Input: dimensioned drawing with shaded views. Units: mm. Origin: part minimum x, y, z. A direction names the side the tool comes from. Round coordinates to 2 decimals unless told otherwise and drop trailing zeros. Loops run counter-clockwise (first coordinate to the right, second up) from the corner with the lowest first, then second, coordinate; pieces in that order, holes last. Notation, with made-up numbers: M 51,-4.5 L 67,-4.5 A15 ccw 67,19.5 Z; hole C -11,-24.75 d6. An arc over 180 degrees is marked long. Return JSON: item names as keys, results as strings.
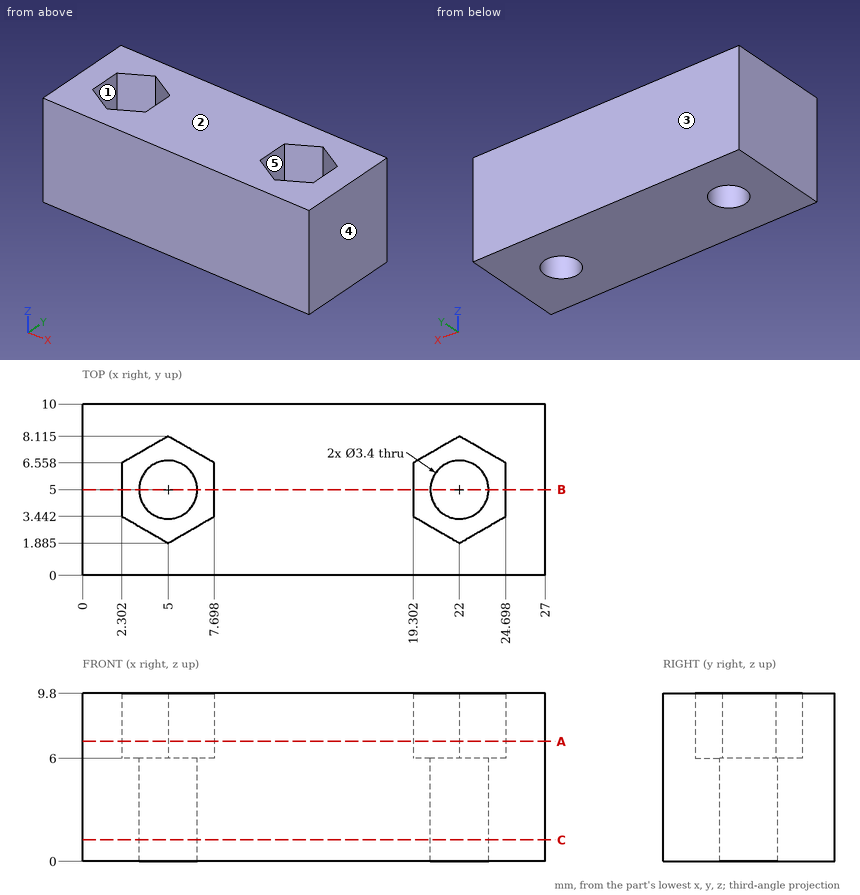
Q1. Material intervals for L1, parallel to X at y = 6, z = 6.75; L2, parallel to Y at x = 22, z = 2.05; L3, parallel to X at y = 5.25, z = 4.5, sorted ascending.
Determined:
{"L1": "x = 0 to 2.3, 7.7 to 19.3, 24.7 to 27", "L2": "y = 0 to 3.3, 6.7 to 10", "L3": "x = 0 to 3.32, 6.68 to 20.32, 23.68 to 27"}
Q2. Section query A-A (z = 7). Output: boundary loops of the cut face in (x, y) (1 decimal).
Determined:
{"outline": "M 0,0 L 27,0 L 27,10 L 0,10 Z; hole M 2.3,3.4 L 5,1.9 L 7.7,3.4 L 7.7,6.6 L 5,8.1 L 2.3,6.6 Z; hole M 19.3,3.4 L 22,1.9 L 24.7,3.4 L 24.7,6.6 L 22,8.1 L 19.3,6.6 Z"}
Q3. Pull-direction query (Y, two-part tool) for the marked faces 1, 2 and 3; classes: pulls with the +Y half, pulls with the -Y half, needs draft (parallel to the pull), parting line crosses it, or undercut.
Determined:
{"face 1": "undercut", "face 2": "needs draft", "face 3": "pulls with the +Y half"}
Q4. Pin query (flat end, axial travel): pin 1 (4 mm diameter, centred on x = 20.5, y = 3.5, fed in from +Z); pin 2 (3 mm diameter, centred on x = 22, y = 5, fed in from +Z); pin 3 (2.5 mm diameter, centred on x = 5, y = 6.5, fed in from +Z). Return the tip coordinate at first contact, or that it passes through.
Determined:
{"pin 1": "stops at z = 9.8", "pin 2": "passes through", "pin 3": "stops at z = 6"}
Q5. Section query B-B (y = 5). Output: boundary loops of the cut face in (x, z).
Determined:
{"outline": "M 0,0 L 3.3,0 L 3.3,6 L 2.3,6 L 2.3,9.8 L 0,9.8 Z; M 6.7,0 L 20.3,0 L 20.3,6 L 19.3,6 L 19.3,9.8 L 7.7,9.8 L 7.7,6 L 6.7,6 Z; M 23.7,0 L 27,0 L 27,9.8 L 24.7,9.8 L 24.7,6 L 23.7,6 Z"}
Q6. Reachability of the marked faces 4 and 5 from +Z, -Z, +X, -X, +Y, -Y: full face, straight path, thin tool, end or side. Return the list, or none.
Determined:
{"face 4": "+Z, -Z, +X, +Y, -Y", "face 5": "+Z"}
Q7. Section query C-C (z = 1.25). Output: boundary loops of the cut face in (x, y), plus the area to 3 significant figures.
Determined:
{"outline": "M 0,0 L 27,0 L 27,10 L 0,10 Z; hole C 5,5 d3.4; hole C 22,5 d3.4", "area": "252 mm^2"}
